Read the model definition and answer for the solid it produces. Units are mm, in the model's axes. A direction names the side the tool comes from. Coordinates: 2 decimals unless noted, no trailing zeros. Loops run counter-clockwise (first coordinate to the right, second up) from the corner with the lowest first, then second, coordinate; pieces in that order, holes last. Notation, with made-up numbers: M 42.25,-7.75 L 71.25,-7.75 A19 ccw 71.25,17.25 Z; hole C 82.5,-36 d4. An arc over 180 degrees is marked long. One line per item, written item: value. Start each with the question number.
Autodesk Inventor part; units mm, degrees
ref_plane "YZ Plane" through (0, 0, 0) normal (1, 0, 0) x (0, 1, 0)
ref_plane "XZ Plane" through (0, 0, 0) normal (0, 1, 0) x (-1, 0, 0)
ref_plane "XY Plane" through (0, 0, 0) normal (0, 0, 1) x (1, 0, 0)
sketch "Sketch1" plane through (0, 0, 0) normal (0, 1, 0) x (-1, 0, 0)
  line L0 (37.3809, 48.8889) -> (-62.6191, 48.8889)
  line L1 (-62.6191, 48.8889) -> (-62.6191, -51.1111)
  line L2 (-62.6191, -51.1111) -> (37.3809, -51.1111)
  line L3 (37.3809, -51.1111) -> (37.3809, 48.8889)
  point P0 (0, 0)
  dimension "d0" = 100
  dimension "d1" = 100
extrude "Extrusion1" add sketch "Sketch1" along normal blind 30
fillet "Fillet1" radius 3 4 edges at (-37.3809, 15, -51.1111) (-37.3809, 15, 48.8889) (62.6191, 15, -51.1111) (62.6191, 15, 48.8889)
shell "Shell1" thickness 3 removed faces 2 at (27.2857, 30, 14.5556) at (27.2857, 0, 14.5556)
sketch "Sketch2" plane through (0, 0, 0) normal (0, -1, 0) x (1, 0, 0)
  line L0 (-34.3809, 48.8889) -> (59.6191, 48.8889)
  line L1 (15.6191, 48.8889) -> (9.6191, 48.8889)
  line L2 (9.6191, 48.8889) -> (9.6191, 29.8889)
  line L3 (9.6191, 29.8889) -> (15.6191, 29.8889)
  line L4 (15.6191, 29.8889) -> (15.6191, 48.8889)
  line L5 (62.6191, 45.8889) -> (62.6191, -48.1111)
  line L6 (62.6191, 1.8889) -> (43.6191, 1.8889)
  line L7 (43.6191, 1.8889) -> (43.6191, -4.1111)
  line L8 (43.6191, -4.1111) -> (62.6191, -4.1111)
  line L9 (62.6191, -4.1111) -> (62.6191, 1.8889)
  line L10 (59.6191, -51.1111) -> (-34.3809, -51.1111)
  line L11 (15.6191, -32.1111) -> (9.6191, -32.1111)
  line L12 (9.6191, -32.1111) -> (9.6191, -51.1111)
  line L13 (9.6191, -51.1111) -> (15.6191, -51.1111)
  line L14 (15.6191, -51.1111) -> (15.6191, -32.1111)
  line L15 (-37.3809, -48.1111) -> (-37.3809, 45.8889)
  line L16 (-18.3809, 1.8889) -> (-37.3809, 1.8889)
  line L17 (-37.3809, 1.8889) -> (-37.3809, -4.1111)
  line L18 (-37.3809, -4.1111) -> (-18.3809, -4.1111)
  line L19 (-18.3809, -4.1111) -> (-18.3809, 1.8889)
  point P0 (0, 0)
  dimension "d6" = 6
  dimension "d7" = 47
  dimension "d8" = 19
  dimension "d9" = 6
  dimension "d10" = 19
  dimension "d11" = 47
  dimension "d12" = 6
  dimension "d13" = 19
  dimension "d14" = 47
  dimension "d15" = 6
  dimension "d16" = 19
  dimension "d17" = 47
extrude "Extrusion2" add sketch "Sketch2" along normal blind 5
sketch "Sketch3" plane through (0, -5, 0) normal (0, -1, 0) x (1, 0, 0)
  line L0 (-34.3809, 48.8889) -> (9.6191, 48.8889)
  line L1 (15.6191, 29.8889) -> (15.6191, 45.8889)
  line L2 (9.6191, 48.8889) -> (15.6191, 48.8889)
  line L3 (15.6191, 48.8889) -> (15.6191, 42.8889)
  line L4 (15.6191, 42.8889) -> (9.6191, 42.8889)
  line L5 (9.6191, 42.8889) -> (9.6191, 48.8889)
  line L6 (-18.3809, 1.8889) -> (-37.3809, 1.8889)
  line L7 (-34.3809, -4.1111) -> (-18.3809, -4.1111)
  line L8 (-37.3809, 1.8889) -> (-31.3809, 1.8889)
  line L9 (-31.3809, 1.8889) -> (-31.3809, -4.1111)
  line L10 (-31.3809, -4.1111) -> (-37.3809, -4.1111)
  line L11 (-37.3809, -4.1111) -> (-37.3809, 1.8889)
  line L12 (9.6191, -32.1111) -> (9.6191, -51.1111)
  line L13 (9.6191, -45.1111) -> (15.6191, -45.1111)
  line L14 (15.6191, -45.1111) -> (15.6191, -51.1111)
  line L15 (15.6191, -51.1111) -> (9.6191, -51.1111)
  line L16 (9.6191, -51.1111) -> (9.6191, -45.1111)
  line L17 (59.6191, 1.8889) -> (43.6191, 1.8889)
  line L18 (62.6191, 45.8889) -> (62.6191, -48.1111)
  line L19 (56.6191, 1.8889) -> (62.6191, 1.8889)
  line L20 (62.6191, 1.8889) -> (62.6191, -4.1111)
  line L21 (62.6191, -4.1111) -> (56.6191, -4.1111)
  line L22 (56.6191, -4.1111) -> (56.6191, 1.8889)
  point P0 (0, 0)
  dimension "d20" = 6
  dimension "d21" = 6
  dimension "d22" = 6
  dimension "d23" = 6
  dimension "d24" = 6
extrude "Extrusion3" add sketch "Sketch3" along normal blind 45
sketch "Sketch4" plane through (0, -50, 0) normal (0, -1, 0) x (1, 0, 0)
  line L0 (15.6191, -48.1111) -> (15.6191, -51.1111)
  line L1 (9.7564, 48.8742) -> (15.6191, 48.8742)
  line L2 (15.6191, -51.1111) -> (9.7564, -51.1111)
  line L3 (-37.3809, 1.8889) -> (-37.3809, 45.8889)
  line L4 (62.6191, 45.8889) -> (62.6191, -48.1111)
  line L5 (62.6191, 1.8889) -> (62.6191, -4.1419)
  line L6 (-37.3809, -4.1419) -> (-37.3809, 1.8889)
  line L7 (-37.3809, 1.8889) -> (9.7564, 1.8889)
  line L8 (15.6191, 1.8889) -> (62.6191, 1.8889)
  line L9 (9.7564, -51.1111) -> (9.7564, -4.1419)
  line L10 (9.7564, 1.8889) -> (9.7564, 48.8742)
  line L11 (62.6191, -4.1419) -> (15.6191, -4.1419)
  line L12 (9.7564, -4.1419) -> (-37.3809, -4.1419)
  line L13 (15.6191, 48.8742) -> (15.6191, 1.8889)
  line L14 (15.6191, -4.1419) -> (15.6191, -51.1111)
  point P0 (0, 0)
extrude "Extrusion4" add sketch "Sketch4" along normal blind 6
properties part number "bottom"
1) Section D-D (y = -29) is taken. Determine the outline of the cut face in (x, z).
2) Flat-ended cylindrical pins translate along their axes: pin 1 (8 mm diameter, centred on y = -15, z = -39.5, fed in from -X); pin 2 (6 mm diameter, centred on x = 8.5, z = 29, fed in from +Y); pin 3 (12 mm diameter, centred on x = 38.5, z = -9, fed in from +Y); pin 4 (4.5 mm diameter, centred on x = 12, y = -54, fed in from +Z). Find the tip coordinate at first contact, or state that the pin passes through.
3) Section C-C (x = 53) is taken. Determine the outline of the cut face in (y, z), then the cut area to 3 significant figures.
4) Consider line 1 along Z through (x, y) = (28.5, 14.5); line 2 along X through (y, z) = (18, -8.5); line 3 along X through (y, z) = (-4.5, -41). Determine where each line is inside the solid, lowest interval first.
5) For a pull along X with two mould halves and no side action, classify faces 5 (the face through (15.619, -34, -47)), 6 (the face through (13, -2, -32.111)), 7 (the face through (-18.381, -2, -1)) as released by +X, released by -X, zero draft, split by the parting line, or undercut.
6) Section A-A (x = -11) is taken. Determine the outline of the cut face in (y, z).
7) A tool of negligible diameter and unlimited length cuts with its end or side. For faces 1 (the face through (43.619, -2, -1)), 2 (the face through (9.756, -53, -28)), 3 (the face through (9.756, -53, 25)), 4 (the face through (13, -5, -39)), from which of +Z, -Z, +X, -X, +Y, -Y can it reach the whole face along a straight path? Write none if from no direction.
8) Section B-B (z = -20) is taken. Determine the outline of the cut face in (x, y).
Results found:
1. outline: M -37.38,-4.11 L -31.38,-4.11 L -31.38,1.89 L -37.38,1.89 Z; M 9.62,-51.11 L 15.62,-51.11 L 15.62,-45.11 L 9.62,-45.11 Z; M 9.62,42.89 L 15.62,42.89 L 15.62,48.89 L 9.62,48.89 Z; M 56.62,-4.11 L 62.62,-4.11 L 62.62,1.89 L 56.62,1.89 Z
2. pin 1: passes through
2. pin 2: stops at y = 0
2. pin 3: stops at y = -50
2. pin 4: stops at z = 48.87
3. outline: M -56,-4.14 L -50,-4.14 L -50,1.89 L -56,1.89 Z; M -5,-4.11 L 0,-4.11 L 0,1.89 L -5,1.89 Z; M 0,-51.11 L 30,-51.11 L 30,-48.11 L 0,-48.11 Z; M 0,45.89 L 30,45.89 L 30,48.89 L 0,48.89 Z
3. area: 246 mm²
4. line 1: z = -51.11 to -48.11, 45.89 to 48.89
4. line 2: x = -37.38 to -34.38, 59.62 to 62.62
4. line 3: x = 9.62 to 15.62
5. face 5: released by +X
5. face 6: zero draft
5. face 7: undercut
6. outline: M -56,-4.14 L -50,-4.14 L -50,1.89 L -56,1.89 Z; M 0,-51.11 L 30,-51.11 L 30,-48.11 L 0,-48.11 Z; M 0,45.89 L 30,45.89 L 30,48.89 L 0,48.89 Z
7. face 1: +Z, -Z, +Y
7. face 2: -Z, -X, -Y
7. face 3: +Z, -X, -Y
7. face 4: +X, -X
8. outline: M -37.38,0 L -34.38,0 L -34.38,30 L -37.38,30 Z; M 9.76,-56 L 15.62,-56 L 15.62,-50 L 9.76,-50 Z; M 59.62,0 L 62.62,0 L 62.62,30 L 59.62,30 Z
